Read the model definition and answer for the solid it produces. Units are mm, in the model's axes. Face numbers are marked on the shaded views. A direction names the side the tool comes from. Round coordinates to 2 decimals unless told otherwise and drop trailing zeros. Order: outer loops, then holes, each group sorted by start corner. A loop starts at its lowest first (then second) coordinate and runs counter-clockwise, first axis right, second up. Notation, with made-up numbers: (54, -39.75) - (109, -39.75) arc R21 ccw to (109, -27.75) - close; hole circle Ø10 at (51, 85.5). An arc over 180 degrees is marked (long way). Answer as a JSON object with one key per item and string values. Group by question number.
Q1. A tool of negligible diameter and unlimited length cuts with its end or side. For the marked faces 5, 6 and 7, from which of +Z, -Z, +X, -X, +Y, -Y can it reach the whole face along a straight path? Write none if from no direction.
Q2. A cutting plane is placed at B-B on z = 1. Determine the outline of the cut face in (x, y).
Q3. A cutting plane is placed at D-D on z = -0.25. Determine the outline of the cut face in (x, y).
Q4. A cutting plane is placed at C-C on y = 78.25. Determine the outline of the cut face in (x, z).
Q5. The mould has two halves that part along Y. Classify the marked faces 1, 2, 3 and 4: pulls with the +Y half, pulls with the -Y half, needs draft (parallel to the pull), parting line crosses it, or undercut.
Q6. A cutting plane is placed at A-A on x = 0. Determine the outline of the cut face in (y, z), and give its area (3 significant figures).
Q7. Consider line 1 (Y direction, x = 0, z = -0.25); line 2 (X direction, y = 79.45, z = 1); line 3 (Y direction, x = 0.75, z = -0.5). Determine where each line is inside the solid, lowest interval first.
Q8. Given pin 1 Ø0.7 at (x, y) = (3.5, 80) entering from -Z; pin 2 Ø2.5 at (x, y) = (-3, 78.5) entering from -Z; pin 3 Ø1.7 at (x, y) = (-0.5, 79) entering from -Z, each flat-ended and moving along its own axis, determine where each tip first touches the part or whether it passes through.
```python
from build123d import *

# Parameters (mm, degrees)
AUFSATZ_LINEAR_START            = 0.5
AUFSATZ_LINEAR_AUSTRAGEN1_DEPTH = 6


with BuildPart() as part:
    # Skizze2 → Aufsatz-Linear austragen1 (new body)
    with BuildSketch(Plane(origin=(0, 75.95, 0), x_dir=(1, 0, 0), z_dir=(0, 1, 0)).offset(AUFSATZ_LINEAR_START)):
        with BuildLine():
            Line((-4.472135955, 0), (-2.193741097, 0))
            ThreePointArc((-2.193741097, 0), (0, 1.75), (2.193741097, 0))
            Line((2.193741097, 0), (4.472135955, 0))
            ThreePointArc((4.472135955, 0), (0, -5), (-4.472135955, 0))
        make_face()
    extrude(amount=AUFSATZ_LINEAR_AUSTRAGEN1_DEPTH)

    # Skizze6 → Schnitt-Rotation4 (revolve, cut)
    with BuildSketch(Plane(origin=(0, 79.45, 0), x_dir=(-1, 0, 0), z_dir=(0, -1, 0))):
        Polygon((-1.7, 0.973940297), (-1.7, -3.026059703), (0, -3.026059703), (0, 1.75), (0, 1.9), (-1.7, 1.9), align=None)
    revolve(axis=Axis((0, 79.45, -1.75), (0, 0, 1)), mode=Mode.SUBTRACT)


solid = part.part
```
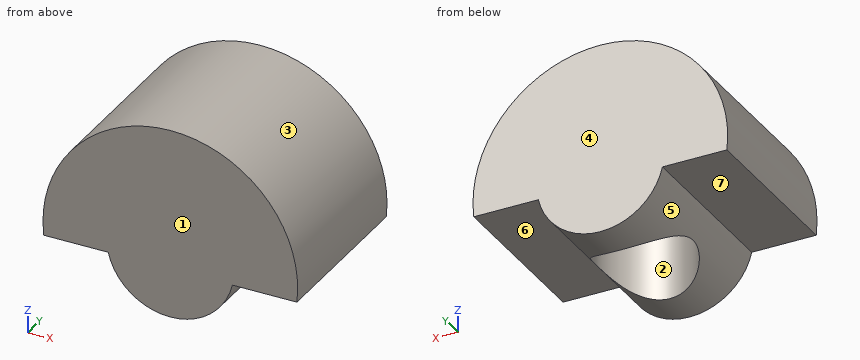
Result set:
{
 "1": {"face 5": "-Z, +Y, -Y", "face 6": "-Z, +X, +Y, -Y", "face 7": "-Z, -X, +Y, -Y"},
 "2": {"outline": "(-4.47, 76.45) - (4.47, 76.45) - (4.47, 82.45) - (-4.47, 82.45) - close; hole circle Ø3.4 at (0, 79.45)"},
 "3": {"outline": "(-2.12, 76.45) - (2.12, 76.45) - (2.12, 82.45) - (-2.12, 82.45) - close; hole circle Ø3.4 at (0, 79.45)"},
 "4": {"outline": "(-4.47, 0) - (-2.19, 0) arc R2.25 ccw to (-1.2, -1.4) - (-1.2, 3.03) - (1.2, 3.03) - (1.2, -1.4) arc R2.25 ccw to (2.19, 0) - (4.47, 0) arc R4.5 ccw (long way) to start"},
 "5": {"face 1": "pulls with the -Y half", "face 2": "undercut", "face 3": "needs draft", "face 4": "pulls with the +Y half"},
 "6": {"outline": "(76.45, -1.75) - (77.75, -1.75) - (77.75, 3.03) - (81.15, 3.03) - (81.15, -1.75) - (82.45, -1.75) - (82.45, 5) - (76.45, 5) - close", "area": "24.3 mm²"},
 "7": {"line 1": "y = 76.45 to 77.75, 81.15 to 82.45", "line 2": "x = -4.47 to -1.7, 1.7 to 4.47", "line 3": "y = 76.45 to 77.92, 80.98 to 82.45"},
 "8": {"pin 1": "stops at z = 0", "pin 2": "stops at z = -0.91", "pin 3": "stops at z = 3.03"}
}
